CAD build for the part. Positions are in the model's coordinates, mm. Face numbers are marked on the shaded views. Give positions to 0.01 mm unless a question says otherwise; leave off trailing zeros. Order: outer loops, then holes, each group sorted by start corner. A loop starts at its lowest first (then second) coordinate and runs counter-clockwise, first axis right, second up.
Autodesk Inventor part; units mm, degrees
ref_plane "YZ Plane" through (0, 0, 0) normal (1, 0, 0) x (0, 1, 0)
ref_plane "XZ Plane" through (0, 0, 0) normal (0, 1, 0) x (-1, 0, 0)
ref_plane "XY Plane" through (0, 0, 0) normal (0, 0, 1) x (1, 0, 0)
sketch "Sketch1" plane through (0, 0, 0) normal (0, 0, 1) x (1, 0, 0)
  line L0 (57.5, -52.5) -> (-57.5, -52.5)
  line L1 (-57.5, -52.5) -> (-57.5, 52.5)
  line L2 (-57.5, 52.5) -> (57.5, 52.5)
  line L3 (57.5, 52.5) -> (57.5, -52.5)
  line L4 (57.5, -52.5) -> (-57.5, 52.5) construction
  line L5 (-57.5, -52.5) -> (57.5, 52.5) construction
  point P0 (0, 0)
  dimension "d0" = 115
  dimension "d1" = 105
extrude "Extrusion1" add sketch "Sketch1" along normal blind 12
fillet "Fillet1" radius 40 2 edges at (-57.5, 52.5, 6) (57.5, 52.5, 6)
sketch "Sketch2" plane through (-57.5, -52.5, 0) normal (0, -1, 0) x (1, 0, 0)
  line L0 (0, 0) -> (0, 12)
  line L1 (115, 0) -> (115, 12)
  line L2 (0, 12) -> (115, 12)
  point P0 (57.5, 0)
  point P1 (10, 6)
  point P2 (105, 6)
  dimension "d5" = 10
  dimension "d6" = 10
  dimension "d7" = 6
  dimension "d8" = 6
hole "Hole1" at (-47.5, -52.5, 6) at (47.5, -52.5, 6) direction (0, 1, 0) diameter 7.134 depth 20.2 tip angle 118
sketch "Sketch3" plane through (0, 0, 12) normal (0, 0, 1) x (1, 0, 0)
  circle A0 centre (0, 0) radius 42.5
  dimension "d16" = 85
extrude "Extrusion2" cut sketch "Sketch3" against normal blind 12
sketch "Sketch4" plane through (0, 0, 12) normal (0, 0, 1) x (1, 0, 0)
  circle A0 centre (0, 0) radius 52.5 construction
  line L0 (0, 0) -> (-64.3477, 64.3477) construction
  line L1 (0, 0) -> (91.0013, 0) construction
  point P0 (-37.1231, 37.1231)
  dimension "d19" = 105
  dimension "d20" = 135
hole "Hole2" at (-37.1231, 37.1231, 12) direction (0, 0, -1) diameter 7.134 depth 20.2 tip angle 118
pattern_circular "Circular Pattern1" count 4 over 360 about axis through (0, 0, -10) along (0, 0, 1) of "Hole2"
properties part number "Gear_support_wheel"
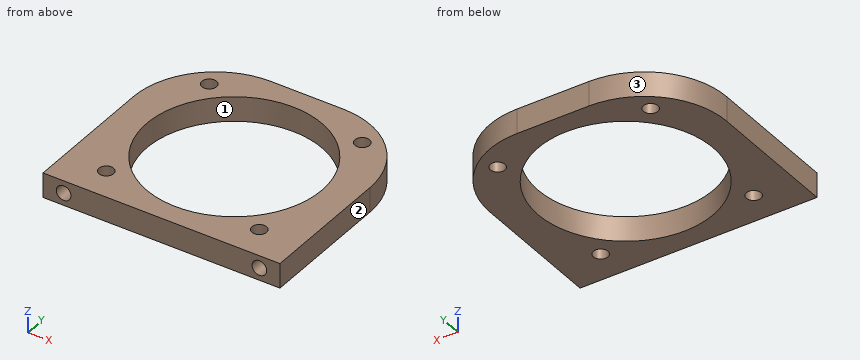
Item 1: Wall check: L1, parallel to X at y = -38.5, z = 6; L2, parallel to Y at x = 36, z = 11; L3, parallel to X at y = 14, z = 7.25. Give the ranges that are in metal, low to high.
Item 2: Slice it at B-B (x = 0). Give the cut face in (y, z).
Item 3: Two-plate mould, pull along Y, no slides. Class the marked faces 1, 2 and 3: released by +Y, released by -Y, zero draft, split by the parting line, or undercut.
Item 4: Drop flat-ended pins along their axis: pin 1 Ø8 at (x, y) = (37.12, 37.12) entering from +Z; pin 2 Ø1.5 at (x, y) = (-4.5, -39.5) entering from -Z; pin 3 Ø1.5 at (x, z) = (36.5, 5.5) entering from +Y; pin 4 Ø6.5 at (x, z) = (47.5, 6) entering from +Y. Give the stop position or say it passes through.
Item 5: Slice it at A-A (y = 0). Give the cut face in (x, z).
Item 6: Slice it at C-C (y = -38.5). Give the cut face in (x, z), and give its area (3 significant figures).
A:
1. L1: x = -57.5 to -51.07, -43.93 to -40.41, -33.83 to -18, 18 to 33.83, 40.41 to 43.93, 51.07 to 57.5
1. L2: y = -52.5 to -40.51, -33.74 to -22.59, 22.59 to 33.74, 40.51 to 47.96
1. L3: x = -57.47 to -40.13, 40.13 to 57.47
2. outline: (-52.5, 0) - (-42.5, 0) - (-42.5, 12) - (-52.5, 12) - close; (42.5, 0) - (52.5, 0) - (52.5, 12) - (42.5, 12) - close
3. face 1: undercut
3. face 2: zero draft
3. face 3: released by +Y
4. pin 1: stops at z = 12
4. pin 2: passes through
4. pin 3: stops at y = 48.09
4. pin 4: stops at y = 42.24
5. outline: (-57.5, 0) - (-42.5, 0) - (-42.5, 12) - (-57.5, 12) - close; (42.5, 0) - (57.5, 0) - (57.5, 12) - (42.5, 12) - close
6. outline: (-57.5, 0) - (-40.41, 0) - (-40.41, 12) - (-57.5, 12) - close; (-33.83, 0) - (-18, 0) - (-18, 12) - (-33.83, 12) - close; (18, 0) - (33.83, 0) - (33.83, 12) - (18, 12) - close; (40.41, 0) - (57.5, 0) - (57.5, 12) - (40.41, 12) - close; hole circle Ø7.13 at (-47.5, 6); hole circle Ø7.13 at (47.5, 6)
6. area: 710 mm2
